Autodesk Inventor part; units mm, degrees
ref_plane "YZ Plane" through (0, 0, 0) normal (1, 0, 0) x (0, 1, 0)
ref_plane "XZ Plane" through (0, 0, 0) normal (0, 1, 0) x (-1, 0, 0)
ref_plane "XY Plane" through (0, 0, 0) normal (0, 0, 1) x (1, 0, 0)
sketch "Sketch1" plane through (0, 0, 0) normal (0, 1, 0) x (-1, 0, 0)
  line L0 (0, 0) -> (38.1, 0)
  line L1 (0, 0) -> (0, -38.1)
  line L2 (0, -38.1) -> (38.1, -38.1)
  line L3 (38.1, -38.1) -> (38.1, 0)
  dimension "d0" = 38.1
  dimension "d2" = 38.1
extrude "Extrusion1" add sketch "Sketch1" along normal blind 38.1
sketch "Sketch2" plane through (0, 38.1, 0) normal (0, 1, 0) x (1, 0, 0)
  circle A0 centre (-19.05, 19.05) radius 19.05
  line L0 (-38.1, 0) -> (-38.1, 38.1)
  line L1 (-38.1, 38.1) -> (0, 38.1)
  point P0 (0, 0)
  dimension "d5" = 19.05
  dimension "d6" = 19.05
  dimension "d7" = 38.1
extrude "Extrusion2" add sketch "Sketch2" along normal blind 82.55 contours A0
sketch "Sketch3" plane through (0, 0, 0) normal (0, -1, 0) x (1, 0, 0)
  circle A0 centre (-19.05, -19.05) radius 6.35
  line L0 (0, -38.1) -> (0, 0)
  line L1 (0, 0) -> (-38.1, 0)
  dimension "d10" = 12.7
  dimension "d11" = 19.05
  dimension "d12" = 19.05
extrude "Extrusion3" add sketch "Sketch3" along normal blind 38.1
properties part number "NeveRest motor"
The listing builds one solid part. Answer for the finished solid, in the listing's coordinates (mm). A direction names the side the tool comes from. Round coordinates to 2 decimals unless told otherwise and drop trailing zeros. Loops run counter-clockwise (first coordinate to the right, second up) from the corner with the lowest first, then second, coordinate; pieces in that order, holes last.
Q1. Section B-B, the plane z = -17 is taken. Determine the outline of the cut face in (x, y).
Q2. Section D-D, the plane x = -22.5 is taken. Determine the outline of the cut face in (y, z) (3 decimals), then the cut area to 3 significant figures.
Q3. Find the intervals of material crossed by line 1 (Y direction, x = -34, z = -23); line 2 (Z direction, x = -19, y = 98.5); line 3 (Z direction, x = -31, y = 77.5), in increasing order.
Q4. Section C-C, the plane y = -15.5 is taken. Determine the outline of the cut face in (x, z), then the cut area to 3 significant figures.
Q5. Given pin 1 Ø4 at (x, y) = (-15.5, 76) entering from -Z; pin 2 Ø10 at (x, y) = (-10, 70.5) entering from +Z; pin 3 Ø1.5 at (x, y) = (-5.5, 80.5) entering from +Z, each flat-ended and moving along its own axis, determine where each tip first touches the part or whether it passes through.
Q6. Which of the six approach directions +Z, -Z, +X, -X, +Y, -Y give full straight-line access (tool end or side, diameter ignored) to faces 1 (the face through (-34.2, 78.8, -30.6)), 2 (the face through (-10, 0, -19)), 3 (the face through (-4, 38.1, -5)), 4 (the face through (-4, 38.1, -33))?
Q7. Section A-A, the plane x = -34.5 is taken. Determine the outline of the cut face in (y, z), then the cut area to 3 significant figures.
Completed:
1. outline: (-38.1, 0) - (-25.06, 0) - (-25.06, -38.1) - (-13.04, -38.1) - (-13.04, 0) - (0, 0) - (0, 38.1) - (-0.11, 38.1) - (-0.11, 120.65) - (-37.99, 120.65) - (-37.99, 38.1) - (-38.1, 38.1) - close
2. outline: (-38.1, -24.381) - (0, -24.381) - (0, -38.1) - (38.1, -38.1) - (38.1, -37.785) - (120.65, -37.785) - (120.65, -0.315) - (38.1, -0.315) - (38.1, 0) - (0, 0) - (0, -13.719) - (-38.1, -13.719) - close
2. area: 4,950 mm2
3. line 1: y = 0 to 120.65
3. line 2: z = -38.1 to 0
3. line 3: z = -33.89 to -4.21
4. outline: circle Ø12.7 at (-19.05, -19.05)
4. area: 127 mm2
5. pin 1: stops at z = -38.04
5. pin 2: stops at z = -0.44
5. pin 3: stops at z = -4.94
6. face 1: +Y
6. face 2: -Y
6. face 3: +Z, +X, +Y
6. face 4: -Z, +X, +Y
7. outline: (0, -38.1) - (38.1, -38.1) - (38.1, -30.19) - (120.65, -30.19) - (120.65, -7.91) - (38.1, -7.91) - (38.1, 0) - (0, 0) - close
7. area: 3,290 mm2
